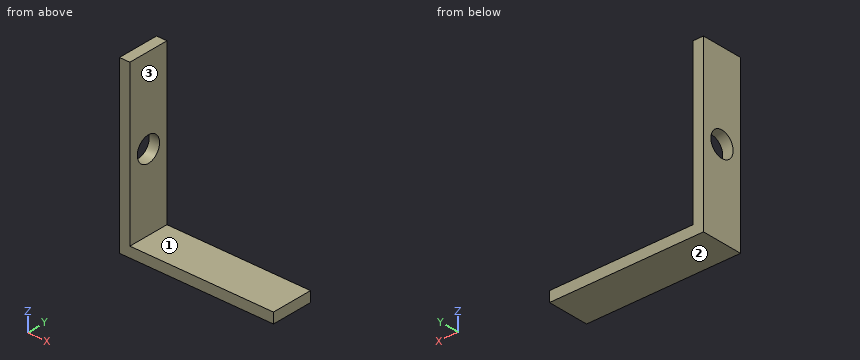
from build123d import *

# Parameters (mm, degrees)
BOSS_EXTRUDE1_DEPTH = 7.9375
SKETCH3_R           = 4.7625
CUT_EXTRUDE1_DEPTH  = 3.96875


with BuildPart() as part:
    # Sketch1 → Boss-Extrude1 (new, symmetric)
    with BuildSketch(Plane(origin=(0, 0, 0), x_dir=(1, 0, 0), z_dir=(0, 1, 0))):
        Polygon((-2.757708096, -19.86108723), (1.211041904, -19.86108723), (1.211041904, 41.25766277), (55.979791904, 41.25766277), (55.979791904, 45.22641277), (6.27967861, 45.22641277), (-2.757708096, 45.22641277), align=None)
    extrude(amount=BOSS_EXTRUDE1_DEPTH, both=True)

    # Sketch3 → Cut-Extrude1 (cut)
    with BuildSketch(Plane.ZY.offset(2.757708096)):
        with Locations((-12.566559842, 0)):
            Circle(SKETCH3_R)
    extrude(amount=-CUT_EXTRUDE1_DEPTH, mode=Mode.SUBTRACT)


solid = part.part
Can you work these out from the model? Positions are in its coordinate system, mm. Face numbers are marked on the shaded views. Give positions to 0.01 mm unless a question says otherwise; leave off trailing zeros. Loops run counter-clockwise (first coordinate to the right, second up) from the corner with the lowest first, then second, coordinate; pieces in that order, holes last. Notation, with made-up numbers: (88.25, 14.5) -> (115.25, 14.5) arc R20 cw to (115.25, 19.5) -> close; hole circle Ø2 at (35, -34). An arc over 180 degrees is marked (long way). Return JSON: item names as keys, results as strings.
Q1. I want a section at D-D, the plane z = -34. List the corners of the cut face in (x, y) for me.
Checks:
{"outline": "(-2.76, -7.94) -> (1.21, -7.94) -> (1.21, 7.94) -> (-2.76, 7.94) -> close"}
Q2. I need wall thicknesses on probe 1 along X at (y, z) = (-2.25, 13.5); probe 2 along Z at (x, y) = (40, -6.5); probe 3 along Z at (x, y) = (0, 0.75). Which ranges of each line are inside material? Lowest first, please.
Checks:
{"probe 1": "x = -2.76 to 1.21", "probe 2": "z = -45.23 to -41.26", "probe 3": "z = -45.23 to -17.27, -7.86 to 19.86"}
Q3. I want a section at B-B, the plane y = 3.25. List the corners of the cut face in (x, z) for me.
Checks:
{"outline": "(-2.76, -45.23) -> (55.98, -45.23) -> (55.98, -41.26) -> (1.21, -41.26) -> (1.21, -16.05) -> (-2.76, -16.05) -> close; (-2.76, -9.09) -> (1.21, -9.09) -> (1.21, 19.86) -> (-2.76, 19.86) -> close"}
Q4. I want a section at C-C, the plane y = 6.5. List the corners of the cut face in (x, z) for me, then the cut area to 3 significant figures.
Checks:
{"outline": "(-2.76, -45.23) -> (55.98, -45.23) -> (55.98, -41.26) -> (1.21, -41.26) -> (1.21, 19.86) -> (-2.76, 19.86) -> close", "area": "476 mm2"}
Q5. I want a section at A-A, the plane y = 0. List the corners of the cut face in (x, z) for me, then the cut area to 3 significant figures.
Checks:
{"outline": "(-2.76, -45.23) -> (55.98, -45.23) -> (55.98, -41.26) -> (1.21, -41.26) -> (1.21, -17.33) -> (-2.76, -17.33) -> close; (-2.76, -7.8) -> (1.21, -7.8) -> (1.21, 19.86) -> (-2.76, 19.86) -> close", "area": "438 mm2"}
Q6. We'd pull the mould along Z, two halves only. Please class the marked faces 1, 2 and 3: released by +Z, released by -Z, zero draft, split by the parting line, or undercut.
Checks:
{"face 1": "released by +Z", "face 2": "released by -Z", "face 3": "zero draft"}
Q7. For pin 1 Ø4 at (y, z) = (-1.5, -10.5) entering from +X; pin 2 Ø3 at (y, z) = (-2.5, -34.5) entering from +X, each with a flat end and sliding along its axis, tell me the tip position at first contact or that it passes through.
Checks:
{"pin 1": "passes through", "pin 2": "stops at x = 1.21"}
